The listing builds one solid part. Answer for the finished solid, in the listing's coordinates (mm). A direction names the side the tool comes from. Round coordinates to 2 decimals unless told otherwise and drop trailing zeros. Order: outer loops, then holes, each group sorted by start corner. A loop starts at its lowest first (then second) coordinate and runs counter-clockwise, first axis right, second up. Notation, with made-up numbers: (42.5, 82) - (99.5, 82) arc R25 ccw to (99.5, 97) - close; hole circle Ø3 at (22.25, -7.5). An arc over 180 degrees is marked (long way). Write item = value, one per line.
from build123d import *

# Parameters (mm, degrees)
BOSS_EXTRUDE1_DEPTH      = 3.175
BOSS_EXTRUDE1_DEPTH_BACK = 0.254
BOSS_EXTRUDE2_DEPTH      = 3.429
LPATTERN1_COUNT          = 8
LPATTERN1_PITCH          = 2.45
FILLET1_R                = 0.3


with BuildPart() as part:
    # Sketch3 → Boss-Extrude1 (new body, two sides)
    with BuildSketch(Plane.XZ) as boss_extrude1_sk:
        with BuildLine():
            ThreePointArc((39.2557, 0), (-17.127226966, 35.322345321), (-24.310512242, -30.822215641))
            Line((-24.310512242, -30.822215641), (-24.310512242, -17.960512242))
            ThreePointArc((-24.310512242, -17.960512242), (-17.960512242, -11.610512242), (-11.610512242, -17.960512242))
            Line((-11.610512242, -17.960512242), (-11.610512242, -37.010512242))
            ThreePointArc((-11.610512242, -37.010512242), (-11.615116608, -37.252285377), (-11.628923029, -37.493707894))
            ThreePointArc((-11.628923029, -37.493707894), (0, -39.2557), (11.628923029, -37.493707894))
            ThreePointArc((11.628923029, -37.493707894), (11.615116608, -37.252285377), (11.610512242, -37.010512242))
            Line((11.610512242, -37.010512242), (11.610512242, -17.960512242))
            ThreePointArc((11.610512242, -17.960512242), (17.960512242, -11.610512242), (24.310512242, -17.960512242))
            Line((24.310512242, -17.960512242), (24.310512242, -30.822215641))
            ThreePointArc((24.310512242, -30.822215641), (35.322345321, -17.127226966), (39.2557, 0))
        make_face()
        with BuildLine():
            ThreePointArc((-5.8, 0), (0, 5.8), (5.8, 0))
            Line((5.8, 0), (5.8, -19.05))
            ThreePointArc((5.8, -19.05), (0, -24.85), (-5.8, -19.05))
            Line((-5.8, -19.05), (-5.8, 0))
        make_face(mode=Mode.SUBTRACT)
        with BuildLine():
            ThreePointArc((-11.590512242, -1.089487758), (-17.960512242, -7.459487758), (-24.330512242, -1.089487758))
            Line((-24.330512242, -1.089487758), (-24.330512242, 17.960512242))
            ThreePointArc((-24.330512242, 17.960512242), (-17.960512242, 24.330512242), (-11.590512242, 17.960512242))
            Line((-11.590512242, 17.960512242), (-11.590512242, -1.089487758))
        make_face(mode=Mode.SUBTRACT)
        with BuildLine():
            ThreePointArc((24.310512242, -1.089487758), (17.960512242, -7.439487758), (11.610512242, -1.089487758))
            Line((11.610512242, -1.089487758), (11.610512242, 17.960512242))
            ThreePointArc((11.610512242, 17.960512242), (17.960512242, 24.310512242), (24.310512242, 17.960512242))
            Line((24.310512242, 17.960512242), (24.310512242, -1.089487758))
        make_face(mode=Mode.SUBTRACT)
    extrude(amount=BOSS_EXTRUDE1_DEPTH)
    extrude(boss_extrude1_sk.sketch, amount=-BOSS_EXTRUDE1_DEPTH_BACK)

    # Sketch4 → Boss-Extrude2 (add)
    with BuildSketch(Plane(origin=(0, 0.254, 0), x_dir=(1, 0, 0), z_dir=(0, 1, 0))):
        Polygon((-5.8, -0.803750085), (-3.94, -0.34), (-3.94, 0.34), (-5.8, 0.803750085), align=None)
    boss_extrude2 = extrude(amount=-BOSS_EXTRUDE2_DEPTH)

    # LPattern1: Boss-Extrude2 ×8
    with Locations(*[(0, 0, -i * LPATTERN1_PITCH) for i in range(1, LPATTERN1_COUNT)]):
        add(boss_extrude2)

    # Fillet1
    fillet1_edges = [part.edges().sort_by_distance(p)[0] for p in [
        (-3.94, -1.4605, 0.34),
        (-5.8, -1.4605, -0.803750085),
        (-3.94, -1.4605, -0.34),
        (-5.7459101, -1.4605, 0.790263959),
        (-5.8, -1.4605, -1.646249915),
        (-5.8, -1.4605, -3.253750085),
        (-3.94, -1.4605, -2.79),
        (-3.94, -1.4605, -2.11),
        (-5.8, -1.4605, -4.096249915),
        (-5.8, -1.4605, -5.703750085),
        (-3.94, -1.4605, -5.24),
        (-3.94, -1.4605, -4.56),
        (-5.8, -1.4605, -6.546249915),
        (-5.8, -1.4605, -8.153750085),
        (-3.94, -1.4605, -7.69),
        (-3.94, -1.4605, -7.01),
        (-5.8, -1.4605, -8.996249915),
        (-5.8, -1.4605, -10.603750085),
        (-3.94, -1.4605, -10.14),
        (-3.94, -1.4605, -9.46),
        (-5.8, -1.4605, -11.446249915),
        (-5.8, -1.4605, -13.053750085),
        (-3.94, -1.4605, -12.59),
        (-3.94, -1.4605, -11.91),
        (-5.8, -1.4605, -13.896249915),
        (-5.8, -1.4605, -15.503750085),
        (-3.94, -1.4605, -15.04),
        (-3.94, -1.4605, -14.36),
        (-5.8, -1.4605, -16.346249915),
        (-5.8, -1.4605, -17.953750085),
        (-3.94, -1.4605, -17.49),
        (-3.94, -1.4605, -16.81),
    ]]
    fillet(fillet1_edges, radius=FILLET1_R)


solid = part.part
Q1. Section D-D on x = 19 is taken. Determine the outline of the cut face in (y, z) (3 decimals), then the cut area to 3 significant figures.
Model answer:
outline = (-3.175, -11.696) - (0.254, -11.696) - (0.254, -7.354) - (-3.175, -7.354) - close; (-3.175, 24.225) - (0.254, 24.225) - (0.254, 34.351) - (-3.175, 34.351) - close
area = 49.6 mm^2
Q2. Determine the mould class of faces 4 (the face through (17.82, -1.48, 24.31)), 5 (the face through (17.821, -1.485, -11.612)), 6 (the face through (-24.311, -1, -24)) for opening direction Z: released by +Z, released by -Z, zero draft, split by the parting line, or undercut.
Model answer:
face_4 = undercut
face_5 = released by -Z
face_6 = zero draft
Q3. Section A-A on x = 0 is taken. Determine the outline of the cut face in (y, z) (3 decimals).
Model answer:
outline = (-3.175, -39.256) - (0.254, -39.256) - (0.254, -24.85) - (-3.175, -24.85) - close; (-3.175, 5.8) - (0.254, 5.8) - (0.254, 39.256) - (-3.175, 39.256) - close
Q4. Find the intervals of material crossed by line 1 (X direction, y = -0.05, z = 23.5); line 2 (X direction, y = -0.8, z = 8); line 3 (X direction, y = -0.95, z = 3.5), in increasing order. Write a range as from..to.
Model answer:
line_1 = -31.44..-21.11, -14.82..14.86, 21.06..31.44
line_2 = -38.43..-24.33, -11.59..11.61, 24.31..38.43
line_3 = -39.1..-24.33, -11.59..-4.62, 4.62..11.61, 24.31..39.1
Q5. Section C-C on y = -2 is taken. Count the separate pieces of the cut face and the enclosed holes in it, then the cut area to 3 significant figures.
Model answer:
separate_pieces = 1
enclosed_holes = 3
area = 3,240 mm^2
Q6. Flat-ended cylindrical pins translate along their axes: P1, Ø1, axis at y = -2, z = -27.5, coming from the -X side; P2, Ø0.9, axis at y = -2, z = -18.5, coming from the +X side; P3, Ø1.7, axis at y = -1, z = -28, coming from the +X side. Find the tip coordinate at first contact, or state that the pin passes through.
Model answer:
P1 = -28.5
P2 = 34.86
P3 = 28.35
Q7. For faces 1 (the face through (-18.1, -1.48, 24.33)), 2 (the face through (8, 0.254, 1)), 3 (the face through (24.311, -1, -24)), determine the directions among +Z, -Z, +X, -X, +Y, -Y from which every point of the face is accessible in a straight line to the end or side of a thin tool.
Model answer:
face_1 = +Y, -Y
face_2 = +Z, -Z, +X, -X, +Y
face_3 = -Z, +Y, -Y
Q8. Section B-B on z = -29 is taken. Determine the outline of the cut face in (x, y) (3 decimals).
Model answer:
outline = (-26.458, -3.175) - (-24.311, -3.175) - (-24.311, 0.254) - (-26.458, 0.254) - close; (-11.611, -3.175) - (11.611, -3.175) - (11.611, 0.254) - (-11.611, 0.254) - close; (24.311, -3.175) - (26.458, -3.175) - (26.458, 0.254) - (24.311, 0.254) - close
